Input: part model. Units: mm. Frame: model coordinates. A direction names the side the tool comes from. Coordinates: 2 decimals unless noted, no trailing zeros. Order: outer loops, then holes, each group sorted by start corner. A loop starts at its lowest first (then second) coordinate and runs counter-clockwise, first axis right, second up. Notation, with made-up numbers: (-6, 74) -> (29, 74) arc R24 ccw to (29, 104) -> close; hole circle Ø4 at (36.5, 53.5). An arc over 180 degrees is marked (long way). One line per question, with ' | ' between items.
Autodesk Inventor part; units mm, degrees
ref_plane "YZ Plane" through (0, 0, 0) normal (1, 0, 0) x (0, 1, 0)
ref_plane "XZ Plane" through (0, 0, 0) normal (0, 1, 0) x (-1, 0, 0)
ref_plane "XY Plane" through (0, 0, 0) normal (0, 0, 1) x (1, 0, 0)
sketch "Sketch1" plane through (0, 0, 0) normal (1, 0, 0) x (0, 1, 0)
  line L0 (0, 0) -> (8.4, 0)
  line L1 (8.4, 0) -> (8.4, 6)
  line L2 (2.4, 12) -> (0, 12)
  arc A0 (8.4, 6) -> (2.4, 12) centre (2.4, 6) ccw
  line L3 (8.4, 0) -> (8.4, -6)
  line L4 (2.4, -12) -> (0, -12)
  arc A1 (2.4, -12) -> (8.4, -6) centre (2.4, -6) ccw
  dimension "d1" = 12
  dimension "d2" = 12
  dimension "d5" = 6
  dimension "d6" = 6
sketch "Sketch2" plane through (0, 0, 0) normal (0, 1, 0) x (-1, 0, 0)
  line L0 (0, 0) -> (0, 12)
  circle A0 centre (0, 12) radius 3.75
  dimension "d7" = 12
  dimension "d8" = 7.5
sweep "Sweep1" add profiles "Sketch2" path "Sketch1" path curves L2 A0 L1 L3 A1 L4
sketch "Sketch3" plane through (0, 0, -12) normal (0, -1, 0) x (1, 0, 0)
  point P0 (0, 12)
properties part number "Tube for ball screew"
1. Cut plane A-A, the plane x = 2.75. Return loops of the section in (y, z).
Recorded:
outline: (0, -14.55) -> (2.4, -14.55) arc R8.55 ccw to (10.95, -6) -> (10.95, 6) arc R8.55 ccw to (2.4, 14.55) -> (0, 14.55) -> (0, 9.45) -> (2.4, 9.45) arc R3.45 cw to (5.85, 6) -> (5.85, -6) arc R3.45 cw to (2.4, -9.45) -> (0, -9.45) -> close
2. Cut plane B-B, the plane z = 0.5. Return loops of the section in (x, y).
Recorded:
outline: circle Ø7.5 at (0, 8.4)
3. Pin query (flat end, axial travel): pin 1 Ø4 at (y, z) = (1, -9) entering from -X; pin 2 Ø1.5 at (x, z) = (1, -11.5) entering from +Y; pin 3 Ø4 at (x, y) = (2, 7.5) entering from -Z. Return the tip coordinate at first contact, or that it passes through.
Recorded:
pin 1: stops at x = -3.61 | pin 2: stops at y = 10.8 | pin 3: stops at z = -15.01
4. Cut plane C-C, the plane x = 0. Return loops of the section in (y, z), and give its area (3 significant figures).
Recorded:
outline: (0, -15.75) -> (2.4, -15.75) arc R9.75 ccw to (12.15, -6) -> (12.15, 6) arc R9.75 ccw to (2.4, 15.75) -> (0, 15.75) -> (0, 8.25) -> (2.4, 8.25) arc R2.25 cw to (4.65, 6) -> (4.65, -6) arc R2.25 cw to (2.4, -8.25) -> (0, -8.25) -> close | area: 267 mm^2
5. Ray query, line 1 (Y direction, x = -3, z = 1.5); line 2 (Z direction, x = -3, y = 4.5); line 3 (Y direction, x = -2.5, z = -4). Return the intervals inside material, ascending. Write a range as [from, to].
Recorded:
line 1: y = [6.15, 10.65] | line 2: z = [-13.98, -9.11], [9.11, 13.98] | line 3: y = [5.6, 11.2]
6. Access query for faces 1 (the face through (3.746, 8.235, 0.084)), 2 (the face through (0, 0, -12)), 3 (the face through (0.488, 1.183, 8.282)). Directions: +Z, -Z, +X, -X, +Y, -Y. A direction counts if a zero-diameter tool reaches every point of the face in a straight line with its end or side. Return the directions, or none.
Recorded:
face 1: none | face 2: +Z, -Z, +X, -X, -Y | face 3: -Y
